Read the model definition and answer for the solid it produces. Units are mm, in the model's axes. Face numbers are marked on the shaded views. A direction names the side the tool comes from. Give positions to 0.01 mm unless a question says otherwise; leave off trailing zeros. Loops run counter-clockwise (first coordinate to the right, second up) from the corner with the lowest first, then second, coordinate; pieces in that order, holes last. Notation, with made-up numbers: (71.5, 36.5) - (118.5, 36.5) arc R7 cw to (118.5, 49.5) - close; hole circle Ø3 at (22.25, 2). An arc over 180 degrees is marked (long way). Write item = value, one per line.
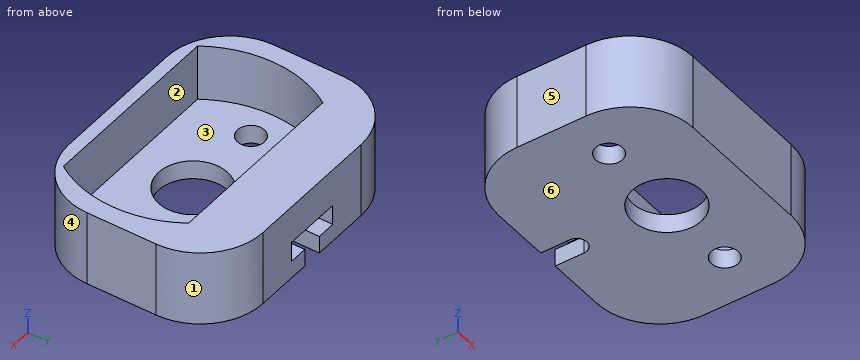
```python
from build123d import *

# Parameters (mm, degrees)
SKETCH1_W               = 42
SKETCH1_H               = 31
BOSS_EXTRUDE1_DEPTH     = 12
CUT_EXTRUDE1_DEPTH      = 9
SKETCH4_R               = 2.15
CUT_EXTRUDE3_DEPTH      = 10
BOSS_EXTRUDE2_START     = -8.28
BOSS_EXTRUDE2_OUTLINE_W = 9.3
BOSS_EXTRUDE2_OUTLINE_H = 3.2
BOSS_EXTRUDE2_DEPTH     = 8.28
SKETCH6_R               = 1.63
CUT_EXTRUDE4_DEPTH      = 2.8
SKETCH7_W               = 3.26
SKETCH7_H               = 4.6
CUT_EXTRUDE5_DEPTH      = 2.8
FILLET1_R               = 10
SKETCH14_R              = 5.5
CUT_EXTRUDE7_DEPTH      = 53.971690553


# Read off the part's stored shape, not the designer's step: Boss-Extrude2
with BuildPart() as part:
    # Sketch1 → Boss-Extrude1 (new body)
    with BuildSketch(Plane.XY):
        with Locations((21, 15.5)):
            Rectangle(SKETCH1_W, SKETCH1_H)
    extrude(amount=BOSS_EXTRUDE1_DEPTH)

    # Sketch2 → Cut-Extrude1 (cut)
    with BuildSketch(Plane.XY.offset(12)):
        with BuildLine():
            Line((36.086749153, 22), (5.913250847, 22))
            ThreePointArc((5.913250847, 22), (2.9, 12), (5.913250847, 2))
            Line((5.913250847, 2), (36.086749153, 2))
            ThreePointArc((36.086749153, 2), (39.1, 12), (36.086749153, 22))
        make_face()
    extrude(amount=-CUT_EXTRUDE1_DEPTH, mode=Mode.SUBTRACT)

    # Sketch4 → Cut-Extrude3 (cut)
    with BuildSketch(Plane.XY.offset(3)):
        with Locations((8, 12)):
            Circle(SKETCH4_R)
        with Locations((34, 12)):
            Circle(SKETCH4_R)
    extrude(amount=-CUT_EXTRUDE3_DEPTH, mode=Mode.SUBTRACT)

    # Boss-Extrude2 outline → Boss-Extrude2 (cut)
    with BuildSketch(Plane(origin=(0, 31, 0), x_dir=(1, 0, 0), z_dir=(0, 1, 0)).offset(BOSS_EXTRUDE2_START)):
        with Locations((21, -4.4)):
            Rectangle(BOSS_EXTRUDE2_OUTLINE_W, BOSS_EXTRUDE2_OUTLINE_H)
    extrude(amount=BOSS_EXTRUDE2_DEPTH, mode=Mode.SUBTRACT)

    # Sketch6 → Cut-Extrude4 (cut)
    with BuildSketch(Plane(origin=(0, 0, 0), x_dir=(-1, 0, 0), z_dir=(0, 0, -1))):
        with Locations((-21, 26.4)):
            Circle(SKETCH6_R)
    extrude(amount=-CUT_EXTRUDE4_DEPTH, mode=Mode.SUBTRACT)

    # Sketch7 → Cut-Extrude5 (cut)
    with BuildSketch(Plane(origin=(0, 0, 0), x_dir=(-1, 0, 0), z_dir=(0, 0, -1))):
        with Locations((-21, 28.7)):
            Rectangle(SKETCH7_W, SKETCH7_H)
    extrude(amount=-CUT_EXTRUDE5_DEPTH, mode=Mode.SUBTRACT)

    # Fillet1
    fillet1_edges = [part.edges().sort_by_distance(p)[0] for p in [
        (0, 0, 6),
        (0, 31, 6),
        (42, 31, 6),
        (42, 0, 6),
    ]]
    fillet(fillet1_edges, radius=FILLET1_R)

    # Sketch14 → Cut-Extrude7 (cut, through all)
    with BuildSketch(Plane.XY.offset(3)):
        with Locations((21, 12)):
            Circle(SKETCH14_R)
    extrude(amount=-CUT_EXTRUDE7_DEPTH, mode=Mode.SUBTRACT)


solid = part.part
```
1) A cutting plane is placed at D-D on x = 30. Determine the outline of the cut face in (y, z), then the cut area to 3 significant figures.
Output:
outline = (0, 0) - (31, 0) - (31, 12) - (22, 12) - (22, 3) - (2, 3) - (2, 12) - (0, 12) - close
area = 192 mm²
2) Find the intervals of material crossed by probe 1 along Z at (x, y) = (17, 28.5); probe 2 along Y at (x, z) = (31, 8); probe 3 along Y at (x, z) = (25.5, 3.5), in increasing order.
Output:
probe_1 = 0 to 2.8, 6 to 12
probe_2 = 0 to 2, 22 to 31
probe_3 = 0 to 2, 22 to 22.72
3) A cutting plane is placed at C-C on y = 12. Determine the outline of the cut face in (x, z), then the cut area to 3 significant figures.
Output:
outline = (0, 0) - (5.85, 0) - (5.85, 3) - (2.9, 3) - (2.9, 12) - (0, 12) - close; (10.15, 0) - (15.5, 0) - (15.5, 3) - (10.15, 3) - close; (26.5, 0) - (31.85, 0) - (31.85, 3) - (26.5, 3) - close; (36.15, 0) - (42, 0) - (42, 12) - (39.1, 12) - (39.1, 3) - (36.15, 3) - close
area = 119 mm²
4) Each of these flat-tipped pins is pushed along its axis until it touches: P1, Ø10, axis at x = 21, y = 14, coming from the +Z side; P2, Ø6, axis at x = 37, z = 5, coming from the -Y side; P3, Ø2.5, axis at y = 25.5, z = 5, coming from the -X side. Where does it stop, or does it pass through?
Output:
P1 = 3
P2 = 0.2
P3 = 0.54
5) The mould has two halves that part along X. Classify the marked faces 3, 4, 5 and 6: pulls with the +X half, pulls with the -X half, needs draft (parallel to the pull), parting line crosses it, or undercut.
Output:
face_3 = undercut
face_4 = pulls with the +X half
face_5 = pulls with the -X half
face_6 = needs draft
6) A tool of negligible diameter and unlimited length cuts with its end or side. For the marked faces 1 and 2, from which of +Z, -Z, +X, -X, +Y, -Y can it reach the whole face along a straight path? Write none if from no direction.
Output:
face_1 = +Z, -Z, +X, +Y
face_2 = +Z
7) A cutting plane is placed at A-A on z = 6.75. Determine the outline of the cut face in (x, y).
Output:
outline = (0, 10) arc R10 ccw to (10, 0) - (32, 0) arc R10 ccw to (42, 10) - (42, 21) arc R10 ccw to (32, 31) - (10, 31) arc R10 ccw to (0, 21) - close; hole (5.91, 2) - (36.09, 2) arc R18.1 ccw to (36.09, 22) - (5.91, 22) arc R18.1 ccw to start
8) A cutting plane is placed at B-B on x = 21. Determine the outline of the cut face in (y, z).
Output:
outline = (0, 0) - (6.5, 0) - (6.5, 3) - (2, 3) - (2, 12) - (0, 12) - close; (17.5, 0) - (24.77, 0) - (24.77, 2.8) - (22.72, 2.8) - (22.72, 6) - (31, 6) - (31, 12) - (22, 12) - (22, 3) - (17.5, 3) - close
